Autodesk Inventor part; units mm, degrees
ref_plane "YZ Plane" through (0, 0, 0) normal (1, 0, 0) x (0, 1, 0)
ref_plane "XZ Plane" through (0, 0, 0) normal (0, 1, 0) x (-1, 0, 0)
ref_plane "XY Plane" through (0, 0, 0) normal (0, 0, 1) x (1, 0, 0)
sketch "草圖1" plane through (0, 0, 0) normal (0, 1, 0) x (-1, 0, 0)
  line L0 (0, 90) -> (9, 90)
  line L1 (9, -90) -> (0, -90)
  line L2 (0, -90) -> (0, 90)
  line L3 (7, 4.5) -> (2, 4.5)
  line L4 (2, 4.5) -> (2, -4.5)
  line L5 (2, -4.5) -> (7, -4.5)
  line L6 (9, 90) -> (9, 100)
  line L7 (9, 100) -> (-6, 100)
  line L8 (-11, 95) -> (-11, 95)
  line L9 (-6, 90) -> (0, 90)
  arc A0 (-11, 95) -> (-6, 90) centre (-6, 95) ccw
  arc A1 (-6, 100) -> (-11, 95) centre (-6, 95) ccw
  circle A2 centre (-6, 95) radius 2.5
  line L10 (9, 0) -> (0, 0)
  line L11 (9, -90) -> (9, -100)
  line L12 (9, -100) -> (-6, -100)
  line L13 (-6, -90) -> (0, -90)
  arc A3 (-6, -90) -> (-11, -95) centre (-6, -95) ccw
  arc A4 (-11, -95) -> (-6, -100) centre (-6, -95) ccw
  circle A5 centre (-6, -95) radius 2.5
  line L14 (9, 90) -> (9, 4.6)
  line L15 (9, -4.6) -> (9, -90)
  line L16 (7, -4.5) -> (7, -4.2)
  line L17 (7, -4.2) -> (9, -4.6)
  line L18 (7, 4.5) -> (7, 4.2)
  line L19 (7, 4.2) -> (9, 4.6)
  point P0 (4.5, 4.5)
  point P1 (4.5, 90)
  point P2 (-11, 100)
  point P3 (-11, -100)
  point P4 (2, 0)
  dimension "d0" = 180
  dimension "d1" = 9
  dimension "d3" = 5
  dimension "d4" = 10
  dimension "d5" = 20
  dimension "d6" = 5
  dimension "d7" = 5
  dimension "d8" = 5
  dimension "d11" = 85.4
  dimension "d12" = 85.4
  dimension "d13" = 9
  dimension "d14" = 0.3
  dimension "d15" = 0.3
  dimension "d16" = 11.31
  dimension "d17" = 0
  dimension "d18" = 5
  dimension "d19" = 20
  dimension "d20" = 185
  dimension "d21" = 20
extrude "擠出1" add sketch "草圖1" along normal blind 3 contours L9 A0 A1 L7 L6 L0 | L0 L14 L19 L18 L3 L4 L10 L2 | L10 L4 L5 L16 L17 L15 L1 L2 | L1 L11 L12 A4 A3 L13 | A2 | A5
properties part number "Lower_Bar_3"
Input: part model. Units: mm. Frame: model coordinates. Coordinates: 2 decimals unless noted, no trailing zeros. Write each loop counter-clockwise with the first axis right and the second up, starting at its lowest first coordinate (ties: lowest second). Pieces come first, ordered by that corner, then holes. Notation, with made-up numbers: (82.5, 53) - (115.5, 53) arc R30 cw to (115.5, 92) - close; hole circle Ø4 at (63, -0.5). An arc over 180 degrees is marked (long way). Put each result on its own line as item: value. Start each with the question number.
1) Mould query, pull axis Z, two halves, no side actions, for faces 1 (the face through (-1, 0, 1)), 2 (the face through (11, 1, -95)). Classes: pulls with the +Z half, pulls with the -Z half, needs draft (parallel to the pull), parting line crosses it, or undercut.
2) Cut plane A-A (x = 4). Return the cut outline in (y, z), plus the area to 3 significant figures.
3) Contact query for flat-ended pins moving along their axis: pin 1 (1.5 mm diameter, centred on y = 1.5, z = 0.5, fed in from -X); pin 2 (0.9 mm diameter, centred on y = 1.5, z = -12, fed in from +X). Output: stop coordinate, or through.
4) Cut plane C-C (z = 13). Return the cut outline in (x, y), plus the area to 3 significant figures.
5) Ray query, L1, parallel to Z at x = -6.5, y = 0.65; L2, parallel to Z at x = 3.5, y = 1.1; L3, parallel to X at y = 2.1, z = -85. Return the intervals inside material, ascending.
6) Cut plane B-B (y = 1.2). Return the cut outline in (x, z), plus the area to 3 significant figures.
Resolved:
1. face 1: needs draft
1. face 2: undercut
2. outline: (0, -100) - (3, -100) - (3, -90) - (0, -90) - close; (0, 90) - (3, 90) - (3, 100) - (0, 100) - close
2. area: 60.0 mm2
3. pin 1: stops at x = -2
3. pin 2: stops at x = 0
4. outline: (-9, 0) - (0, 0) - (0, 3) - (-9, 3) - close
4. area: 27.0 mm2
5. L1: z = -100 to -4.5, 4.5 to 100
5. L2: z = -100 to -90, 90 to 100
5. L3: x = -9 to 0
6. outline: (-9, -100) - (6, -100) arc R5 ccw to (6, -90) - (0, -90) - (0, 90) - (6, 90) arc R5 ccw to (6, 100) - (-9, 100) - (-9, 4.6) - (-7, 4.2) - (-7, 4.5) - (-2, 4.5) - (-2, -4.5) - (-7, -4.5) - (-7, -4.2) - (-9, -4.6) - close
6. area: 1,940 mm2
